```python
from build123d import *

# Parameters (mm, degrees)
SKETCH1_R               = 9.7
BOSS_EXTRUDE1_DEPTH     = 5.35
SKETCH2_R               = 9.7
SKETCH2_R_2             = 8.65
CUT_EXTRUDE1_DEPTH      = 1.95
SKETCH3_R               = 9.7
SKETCH3_R_2             = 8.65
CUT_EXTRUDE2_DEPTH      = 1.95
CUT_EXTRUDE3_DEPTH      = 2.95
CUT_EXTRUDE3_DEPTH_BACK = 1.95
SKETCH5_R               = 7.99
CUT_EXTRUDE4_DEPTH      = 6.35
CUT_EXTRUDE5_DEPTH      = 10.7
CIRPATTERN1_COUNT       = 3


with BuildPart() as part:
    # Sketch1 → Boss-Extrude1 (new body)
    with BuildSketch(Plane(origin=(0, 0, 0), x_dir=(1, 0, 0), z_dir=(0, 1, 0))):
        Circle(SKETCH1_R)
    extrude(amount=BOSS_EXTRUDE1_DEPTH)

    # Sketch2 → Cut-Extrude1 (cut)
    with BuildSketch(Plane(origin=(0, 5.35, 0), x_dir=(1, 0, 0), z_dir=(0, 1, 0))):
        Circle(SKETCH2_R)
        Circle(SKETCH2_R_2, mode=Mode.SUBTRACT)
    extrude(amount=-CUT_EXTRUDE1_DEPTH, mode=Mode.SUBTRACT)

    # Sketch3 → Cut-Extrude2 (cut)
    with BuildSketch(Plane.XZ):
        Circle(SKETCH3_R)
        Circle(SKETCH3_R_2, mode=Mode.SUBTRACT)
    extrude(amount=-CUT_EXTRUDE2_DEPTH, mode=Mode.SUBTRACT)

    # Sketch4 → Cut-Extrude3 (cut, two sides)
    with BuildSketch(Plane(origin=(0, 3.4, 0), x_dir=(1, 0, 0), z_dir=(0, 1, 0))) as cut_extrude3_sk:
        with BuildLine():
            Line((-35.407684365, 52.835510073), (-1.8, 9.531526635))
            ThreePointArc((-1.8, 9.531526635), (0, 8.65), (1.8, 9.531526635))
            Line((1.8, 9.531526635), (35.407684365, 52.835510073))
            Line((35.407684365, 52.835510073), (35.407684365, 162.466006376))
            Line((35.407684365, 162.466006376), (-35.407684365, 162.466006376))
            Line((-35.407684365, 162.466006376), (-35.407684365, 52.835510073))
        make_face()
    extrude(amount=CUT_EXTRUDE3_DEPTH, mode=Mode.SUBTRACT)
    extrude(cut_extrude3_sk.sketch, amount=-CUT_EXTRUDE3_DEPTH_BACK, mode=Mode.SUBTRACT)

    # Sketch5 → Cut-Extrude4 (cut, through all)
    with BuildSketch(Plane(origin=(0, 5.35, 0), x_dir=(1, 0, 0), z_dir=(0, 1, 0))):
        Circle(SKETCH5_R)
    extrude(amount=-CUT_EXTRUDE4_DEPTH, mode=Mode.SUBTRACT)

    # Sketch6 → Cut-Extrude5 (cut, through all)
    with BuildSketch(Plane.XY):
        Polygon((0, 3.4), (-2.06, 3.4), (-2.58, 5.35), (0, 5.35), (2.58, 5.35), (2.06, 3.4), align=None)
    cut_extrude5 = extrude(amount=CUT_EXTRUDE5_DEPTH, mode=Mode.SUBTRACT)

    # CirPattern1: Cut-Extrude5 ×3 about axis
    cirpattern1_axis = Axis((0, 0, 0), (0, 1, 0))
    for i in range(1, CIRPATTERN1_COUNT):
        add(cut_extrude5.rotate(cirpattern1_axis, i * 360 / CIRPATTERN1_COUNT), mode=Mode.SUBTRACT)


solid = part.part
```
Input: part model. Units: mm. Frame: model coordinates. A direction names the side the tool comes from. Give positions to 0.01 mm unless a question says otherwise; leave off trailing zeros. Order: outer loops, then holes, each group sorted by start corner. A loop starts at its lowest first (then second) coordinate and runs counter-clockwise, first axis right, second up. Notation, with made-up numbers: (89.5, 40) - (102.5, 40) arc R16 ccw to (102.5, 54) - close; hole circle Ø3 at (40, 85). An arc over 180 degrees is marked (long way). Use a Markdown table: item, result.
(1) Line query: line 1 (X direction, y = 2.75, z = 0); line 2 (Z direction, x = 0, y = 1.6); line 3 (Z direction, x = 0, y = 2.8). Output: solid intervals per line, ascending. Write a range as from..to.
Computed values:
| item | result |
|---|---|
| line 1 | x = -9.7..-7.99, 7.99..9.7 |
| line 2 | z = -8.65..-7.99, 7.99..8.65 |
| line 3 | z = -8.65..-7.99, 7.99..9.7 |
(2) Section query C-C (x = 3.25). Output: boundary loops of the cut face in (y, z), then the cut area to 3 significant figures.
Computed values:
| item | result |
|---|---|
| outline | (0, -8.02) - (1.95, -8.02) - (1.95, -9.14) - (3.4, -9.14) - (3.4, -8.02) - (5.35, -8.02) - (5.35, -7.3) - (0, -7.3) - close; (0, 7.3) - (5.35, 7.3) - (5.35, 8.02) - (3.4, 8.02) - (3.4, 9.14) - (1.95, 9.14) - (1.95, 8.02) - (0, 8.02) - close |
| area | 10.9 mm2 |
(3) Section query A-A (z = 0). Output: boundary loops of the cut face in (x, y), then the cut area to 3 significant figures.
Computed values:
| item | result |
|---|---|
| outline | (-9.7, 1.95) - (-8.65, 1.95) - (-8.65, 0) - (-7.99, 0) - (-7.99, 5.35) - (-8.65, 5.35) - (-8.65, 3.4) - (-9.7, 3.4) - close; (7.99, 0) - (8.65, 0) - (8.65, 1.95) - (9.7, 1.95) - (9.7, 3.4) - (8.65, 3.4) - (8.65, 5.35) - (7.99, 5.35) - close |
| area | 10.1 mm2 |
(4) Section query B-B (y = 4.9). Output: boundary loops of the cut face in (x, z).
Computed values:
| item | result |
|---|---|
| outline | (-8.41, -2.02) - (-7.81, -1.67) arc R7.99 cw to (-2.46, 7.6) - (-2.46, 8.29) arc R8.65 ccw to start; (-5.95, -6.28) arc R8.65 ccw to (5.95, -6.28) - (5.35, -5.93) arc R7.99 cw to (-5.35, -5.93) - close; (2.46, 7.6) arc R7.99 cw to (7.81, -1.67) - (8.41, -2.02) arc R8.65 ccw to (2.46, 8.29) - close |
(5) Draft query along Z for faces 1 (the flat face through (2.324, 4.389, 7.976)), 2 (the flat face through (-5.749, 4.361, -5.994)), 3 (the flat face through (-8.069, 4.389, -1.976)), 4 (the flat face through (5.745, 4.389, -6)). Return one class per face: released by +Z, released by -Z, zero draft, split by the parting line, or undercut.
Computed values:
| item | result |
|---|---|
| face 1 | zero draft |
| face 2 | undercut |
| face 3 | released by -Z |
| face 4 | undercut |
(6) Access query for faces 5 (the flat face through (-7, 3.4, 6)), 6 (the flat face through (-2.316, 4.361, 7.976)), 7 (the cylindrical face through (0.1, 4.39, -8.65)), 8 (the cylindrical face through (7.44, 4.39, 4.41)), 9 (the cylindrical face through (8.25, 0.96, 2.6)). Directions: +Z, -Z, +X, -X, +Y, -Y. A direction counts if a zero-diameter tool reaches every point of the face in a straight line with its end or side. Return the directions, or none.
Computed values:
| item | result |
|---|---|
| face 5 | +Y |
| face 6 | +Z, +Y |
| face 7 | -Z, +Y |
| face 8 | +X, +Y |
| face 9 | -Y |
(7) Section query D-D (z = -3). Output: boundary loops of the cut face in (x, y).
Computed values:
| item | result |
|---|---|
| outline | (-9.22, 1.95) - (-8.11, 1.95) - (-8.11, 0) - (-7.41, 0) - (-7.41, 3.4) - (-9.22, 3.4) - close; (7.41, 0) - (8.11, 0) - (8.11, 1.95) - (9.22, 1.95) - (9.22, 3.4) - (7.41, 3.4) - close |
(8) Pin query (flat end, axial travel): pin 1 (2 mm diameter, centred on x = -4, y = 2, fed in from -Z). Return the tip coordinate at first contact, or that it passes through.
Computed values:
| item | result |
|---|---|
| pin 1 | stops at z = -9.22 |
